```python
from build123d import *

# Parameters (mm, degrees)
SKETCH2_W           = 139.7
SKETCH2_H           = 254
BASE_FLANGE1_DEPTH  = 0.7
EDGE_FLANGE4_DEPTH  = 139.7
EDGE_FLANGE5_DEPTH  = 255
EDGE_FLANGE6_DEPTH  = 255
EDGE_FLANGE7_DEPTH  = 25.4
EDGE_FLANGE9_DEPTH  = 25.4
EDGE_FLANGE10_DEPTH = 101.6
EDGE_FLANGE11_DEPTH = 101.6
SKETCH76_W          = 12.7
SKETCH76_H          = 12.7
TAB1_DEPTH          = 0.7
SKETCH79_W          = 12.7
SKETCH79_H          = 12.7
TAB2_DEPTH          = 0.7
SKETCH86_R          = 3.15
CUT_EXTRUDE3_DEPTH  = 286.615738362


# Sheet-metal steps are written as plain solids
with BuildPart() as part:
    # Sketch2 → Base-Flange1 (new body)
    with BuildSketch(Plane(origin=(0, 0, 0), x_dir=(1, 0, 0), z_dir=(0, 1, 0))):
        Rectangle(SKETCH2_W, SKETCH2_H)
    extrude(amount=-BASE_FLANGE1_DEPTH)

    # Edge-Flange4 section (across the edge) → Edge-Flange4 (add)
    with BuildSketch(Plane(origin=(69.85, 0, -129), x_dir=(0, 0, 1), z_dir=(-1, 0, 0))):
        with BuildLine():
            Line((-0.7, 1), (-0.7, 202.5))
            Line((-0.7, 202.5), (0, 202.5))
            Line((0, 202.5), (0, 1))
            ThreePointArc((0, 1), (0.292893219, 0.292893219), (1, 0))
            Line((1, 0), (2, 0))
            Line((2, 0), (2, -0.7))
            Line((2, -0.7), (1, -0.7))
            ThreePointArc((1, -0.7), (-0.202081528, -0.202081528), (-0.7, 1))
        make_face()
    extrude(amount=EDGE_FLANGE4_DEPTH)

    # Edge-Flange5 section (across the edge) → Edge-Flange5 (add)
    with BuildSketch(Plane(origin=(-71.85, 0, -128), x_dir=(1, 0, 0), z_dir=(0, 0, 1))):
        with BuildLine():
            Line((-0.7, 1), (-0.7, 202.5))
            Line((-0.7, 202.5), (0, 202.5))
            Line((0, 202.5), (0, 1))
            ThreePointArc((0, 1), (0.292893219, 0.292893219), (1, 0))
            Line((1, 0), (2, 0))
            Line((2, 0), (2, -0.7))
            Line((2, -0.7), (1, -0.7))
            ThreePointArc((1, -0.7), (-0.202081528, -0.202081528), (-0.7, 1))
        make_face()
    extrude(amount=EDGE_FLANGE5_DEPTH)

    # Edge-Flange6 section (across the edge) → Edge-Flange6 (add)
    with BuildSketch(Plane(origin=(71.85, 0, 127), x_dir=(-1, 0, 0), z_dir=(0, 0, -1))):
        with BuildLine():
            Line((-0.7, 1), (-0.7, 202.5))
            Line((-0.7, 202.5), (0, 202.5))
            Line((0, 202.5), (0, 1))
            ThreePointArc((0, 1), (0.292893219, 0.292893219), (1, 0))
            Line((1, 0), (2, 0))
            Line((2, 0), (2, -0.7))
            Line((2, -0.7), (1, -0.7))
            ThreePointArc((1, -0.7), (-0.202081528, -0.202081528), (-0.7, 1))
        make_face()
    extrude(amount=EDGE_FLANGE6_DEPTH)

    # Edge-Flange7 section (across the edge) → Edge-Flange7 (add)
    with BuildSketch(Plane(origin=(-71.85, 151.7, -129.8), x_dir=(0, 0, 1), z_dir=(0, 1, 0))):
        with BuildLine():
            Line((-0.7, 1), (-0.7, 24.7))
            Line((-0.7, 24.7), (0, 24.7))
            Line((0, 24.7), (0, 1))
            ThreePointArc((0, 1), (0.292893219, 0.292893219), (1, 0))
            Line((1, 0), (1.8, 0))
            Line((1.8, 0), (1.8, -0.7))
            Line((1.8, -0.7), (1, -0.7))
            ThreePointArc((1, -0.7), (-0.202081528, -0.202081528), (-0.7, 1))
        make_face()
    extrude(amount=EDGE_FLANGE7_DEPTH)

    # Edge-Flange9 section (across the edge) → Edge-Flange9 (add)
    with BuildSketch(Plane(origin=(71.85, 177.1, -129.8), x_dir=(0, 0, 1), z_dir=(0, -1, 0))):
        with BuildLine():
            Line((-0.7, 1), (-0.7, 24.7))
            Line((-0.7, 24.7), (0, 24.7))
            Line((0, 24.7), (0, 1))
            ThreePointArc((0, 1), (0.292893219, 0.292893219), (1, 0))
            Line((1, 0), (1.8, 0))
            Line((1.8, 0), (1.8, -0.7))
            Line((1.8, -0.7), (1, -0.7))
            ThreePointArc((1, -0.7), (-0.202081528, -0.202081528), (-0.7, 1))
        make_face()
    extrude(amount=EDGE_FLANGE9_DEPTH)

    # Edge-Flange10 section (across the edge) → Edge-Flange10 (add)
    with BuildSketch(Plane(origin=(71.85, 75.5, 128.8), x_dir=(0, 0, -1), z_dir=(0, 1, 0))):
        with BuildLine():
            Line((-0.7, 1), (-0.7, 10))
            Line((-0.7, 10), (0, 10))
            Line((0, 10), (0, 1))
            ThreePointArc((0, 1), (0.292893219, 0.292893219), (1, 0))
            Line((1, 0), (1.8, 0))
            Line((1.8, 0), (1.8, -0.7))
            Line((1.8, -0.7), (1, -0.7))
            ThreePointArc((1, -0.7), (-0.202081528, -0.202081528), (-0.7, 1))
        make_face()
    extrude(amount=EDGE_FLANGE10_DEPTH)

    # Edge-Flange11 section (across the edge) → Edge-Flange11 (add)
    with BuildSketch(Plane(origin=(-71.85, 177.1, 128.8), x_dir=(0, 0, -1), z_dir=(0, -1, 0))):
        with BuildLine():
            Line((-0.7, 1), (-0.7, 10))
            Line((-0.7, 10), (0, 10))
            Line((0, 10), (0, 1))
            ThreePointArc((0, 1), (0.292893219, 0.292893219), (1, 0))
            Line((1, 0), (1.8, 0))
            Line((1.8, 0), (1.8, -0.7))
            Line((1.8, -0.7), (1, -0.7))
            ThreePointArc((1, -0.7), (-0.202081528, -0.202081528), (-0.7, 1))
        make_face()
    extrude(amount=EDGE_FLANGE11_DEPTH)

    # Sketch76 → Tab1 (add)
    with BuildSketch(Plane.ZY.offset(72.55)):
        with Locations((133.35, 8.35)):
            Rectangle(SKETCH76_W, SKETCH76_H)
    extrude(amount=-TAB1_DEPTH)

    # Sketch79 → Tab2 (add)
    with BuildSketch(Plane(origin=(72.55, 0, 0), x_dir=(0, 0, -1), z_dir=(1, 0, 0))):
        with Locations((-133.35, 8.35)):
            Rectangle(SKETCH79_W, SKETCH79_H)
    extrude(amount=-TAB2_DEPTH)

    # Sketch86 → Cut-Extrude3 (cut, through all)
    with BuildSketch(Plane(origin=(72.55, 0, 0), x_dir=(0, 0, -1), z_dir=(1, 0, 0))):
        with Locations(Location((-133.35, 8.35, 0), (0, 0, 90))):
            Circle(SKETCH86_R)
    extrude(amount=-CUT_EXTRUDE3_DEPTH, mode=Mode.SUBTRACT)


solid = part.part
```
Design review of the part built by this model. Coordinates are the model's own, in mm. A direction names the side the tool comes from. Coordinates: 2 decimals unless noted, no trailing zeros. Loops run counter-clockwise (first coordinate to the right, second up) from the corner with the lowest first, then second, coordinate; pieces in that order, holes last. Notation, with made-up numbers: (56.25, 40) -> (89.25, 40) arc R15 cw to (89.25, 55) -> close; hole circle Ø3 at (83.5, 69). An arc over 180 degrees is marked (long way). Answer as a JSON object with one key per item and string values.
Q1. To check wall thickness, follow L1, parallel to Z at x = 72.4, y = 8.35; L2, parallel to X at y = 178, z = 57.5; L3, parallel to Y at x = 72.05, z = 133.35. State the ranges of each line that lie inside material, in increasing order.
Answer block:
{"L1": "z = -128 to 130.2, 136.5 to 139.7", "L2": "x = -72.55 to -71.85, 71.85 to 72.55", "L3": "y = 2 to 5.2, 11.5 to 14.7"}
Q2. Tool access review of faces 4 (the flat face through (-66, 127, 128.8)), 5 (the flat face through (59, 165, -130.5)), 6 (the flat face through (1, 0, 1)): name each direction out of +Z, -Z, +X, -X, +Y, -Y from which nothing blocks a thin tool from reaching the whole face with its end or side.
Answer block:
{"face 4": "+Y, -Y", "face 5": "-Z, +X, -X, +Y, -Y", "face 6": "+Z, +Y"}
Q3. Take a section at C-C on y = 8.35. Give the boundary of the cut face in (x, z).
Answer block:
{"outline": "(-72.55, -128) -> (-71.85, -128) -> (-71.85, 130.2) -> (-72.55, 130.2) -> close; (-72.55, 136.5) -> (-71.85, 136.5) -> (-71.85, 139.7) -> (-72.55, 139.7) -> close; (-69.85, -129.7) -> (69.85, -129.7) -> (69.85, -129) -> (-69.85, -129) -> close; (71.85, -128) -> (72.55, -128) -> (72.55, 130.2) -> (71.85, 130.2) -> close; (71.85, 136.5) -> (72.55, 136.5) -> (72.55, 139.7) -> (71.85, 139.7) -> close"}
Q4. Take a section at B-B on y = 100.5. Give the boundary of the cut face in (x, z).
Answer block:
{"outline": "(-72.55, -128) -> (-71.85, -128) -> (-71.85, 127.8) arc R1 cw to (-70.85, 128.8) -> (-61.85, 128.8) -> (-61.85, 129.5) -> (-70.85, 129.5) arc R1.7 ccw to (-72.55, 127.8) -> close; (-69.85, -129.7) -> (69.85, -129.7) -> (69.85, -129) -> (-69.85, -129) -> close; (61.85, 128.8) -> (70.85, 128.8) arc R1 cw to (71.85, 127.8) -> (71.85, -128) -> (72.55, -128) -> (72.55, 127.8) arc R1.7 ccw to (70.85, 129.5) -> (61.85, 129.5) -> close"}
Q5. Take a section at D-D on x = 21.5. Give the boundary of the cut face in (y, z), plus the area to 3 significant figures.
Answer block:
{"outline": "(-0.7, -128) arc R1.7 ccw to (1, -129.7) -> (202.5, -129.7) -> (202.5, -129) -> (1, -129) arc R1 cw to (0, -128) -> (0, 127) -> (-0.7, 127) -> close", "area": "321 mm^2"}
Q6. Take a section at A-A on z = 133.35. Give the boundary of the cut face in (x, y).
Answer block:
{"outline": "(-72.55, 2) -> (-71.85, 2) -> (-71.85, 5.2) -> (-72.55, 5.2) -> close; (-72.55, 11.5) -> (-71.85, 11.5) -> (-71.85, 14.7) -> (-72.55, 14.7) -> close; (71.85, 2) -> (72.55, 2) -> (72.55, 5.2) -> (71.85, 5.2) -> close; (71.85, 11.5) -> (72.55, 11.5) -> (72.55, 14.7) -> (71.85, 14.7) -> close"}
Q7. Clearance check with flat-ended pins moving along their axes: pin 1 Ø2 at (x, z) = (67, 128) entering from +Y; pin 2 Ø12 at (x, y) = (-46, 26.5) entering from +Z; pin 3 Ø0.6 at (y, z) = (163.5, -130.5) entering from +X. State where each tip first meets the part, or that it passes through.
Answer block:
{"pin 1": "stops at y = 177.1", "pin 2": "stops at z = -129", "pin 3": "stops at x = 71.81"}
Q8. The part is to be moulded in two halves that separate along X. For faces 1 (the flat face through (72.55, 100, 7)), 2 (the flat face through (-71.85, 103, 4)), 3 (the cylindrical face through (-72.195, 7.94, 136.473)), say which applies: +X half, -X half, draft (parallel to the pull), parting line (faces both ways), or undercut.
Answer block:
{"face 1": "+X half", "face 2": "undercut", "face 3": "draft"}
